Work out the finished part from the listing and answer in its coordinate system (mm). Face numbers are marked on the shaded views. A direction names the side the tool comes from. Give positions to 0.01 mm unless a question says otherwise; leave off trailing zeros. Order: outer loops, then holes, each group sorted by start corner. A loop starts at its lowest first (then second) coordinate and runs counter-clockwise, first axis right, second up. Notation, with made-up numbers: M -17.75,41.25 L 40.25,41.25 A20 cw 40.25,64.25 Z; hole C 44,-31 d2. An arc over 180 degrees is marked long. One line per item, written item: value.
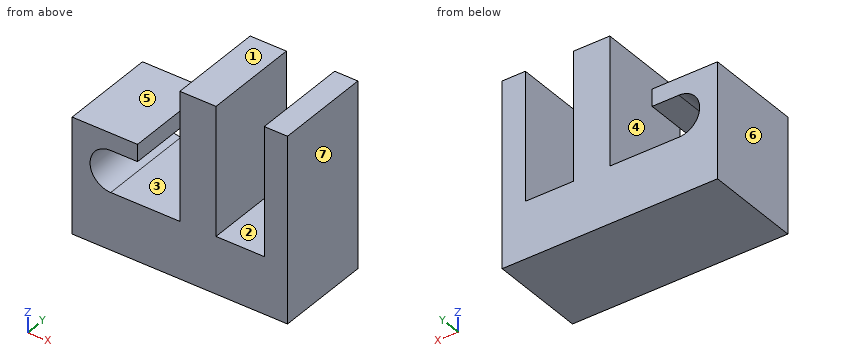
from build123d import *

# Parameters (mm, degrees)
F0_W     = 24.481366
F0_H     = 135.034486
F0_W_2   = 38.1
F0_W_3   = 40.646148
F0_H_2   = 59.899588
F0_H_3   = 43.641134
F0_H_4   = 17.969872
F0_W_4   = 28.23838
F1_DEPTH = 50.8
F3_DEPTH = 176.784


with BuildPart() as f1:
    # F0 (on Front) → F1 (new body, symmetric)
    with BuildSketch(Plane.XZ):
        with Locations((101.140683, 97.467037)):
            Rectangle(F0_W, F0_H)
        with Locations((19.05, 97.467037)):
            Rectangle(F0_W_2, F0_H)
        Polygon((38.1, 29.949794), (0, 29.949794), (-72.735218, 29.949794), (-72.735218, -29.949794), (113.381366, -29.949794), (113.381366, 29.949794), (88.9, 29.949794), align=None)
        with Locations((-93.058292, 0)):
            Rectangle(F0_W_3, F0_H_2)
        with Locations((-93.058292, 51.770361)):
            Rectangle(F0_W_3, F0_H_3)
        with Locations((-93.058292, 82.575864)):
            Rectangle(F0_W_3, F0_H_4)
        with Locations((-58.616028, 82.575864)):
            Rectangle(F0_W_4, F0_H_4)
    extrude(amount=F1_DEPTH, both=True)

    # F2 (on face) → F3 (cut)
    with BuildSketch(Plane.XZ.offset(50.8)):
        with BuildLine():
            Line((-72.735218, 29.949794), (-72.735218, 73.590928))
            ThreePointArc((-72.735218, 73.590928), (-94.555785, 51.770361), (-72.735218, 29.949794))
        make_face()
    extrude(amount=-F3_DEPTH, mode=Mode.SUBTRACT)


solid = f1.part
(1) Section B-B, the plane z = 153 is taken. Give the vertices of the cut face in (x, y).
Findings:
outline: M 0,-50.8 L 38.1,-50.8 L 38.1,50.8 L 0,50.8 Z; M 88.9,-50.8 L 113.38,-50.8 L 113.38,50.8 L 88.9,50.8 Z
(2) Determine the mould class of the marked faces 4, 5, 6 and 7 for opening direction X: pulls with the +X half, pulls with the -X half, needs draft (parallel to the pull), parting line crosses it, or undercut.
Findings:
face 4: undercut
face 5: needs draft
face 6: pulls with the -X half
face 7: pulls with the +X half
(3) Given P1, Ø1.5, axis at x = -26, y = -11, coming from the +Z side, flat-ended and moving along its own axis, determine where the tip first touches the part or whether it passes through.
Findings:
P1: stops at z = 29.95
(4) Find the intervals of material crossed by probe 1 along X at (y, z) = (-37.5, 156.5); probe 2 along X at (y, z) = (-37, 84.5); probe 3 along X at (y, z) = (-9.5, 49.5), in increasing order. Write a range as from..to.
Findings:
probe 1: x = 0..38.1, 88.9..113.38
probe 2: x = -113.38..-44.5, 0..38.1, 88.9..113.38
probe 3: x = -113.38..-94.44, 0..38.1, 88.9..113.38
(5) Section D-D, the plane y = 37.5 is taken. Give the vertices of the cut face in (x, z).
Findings:
outline: M -113.38,-29.95 L 113.38,-29.95 L 113.38,164.98 L 88.9,164.98 L 88.9,29.95 L 38.1,29.95 L 38.1,164.98 L 0,164.98 L 0,29.95 L -72.74,29.95 A21.82 cw -72.74,73.59 L -44.5,73.59 L -44.5,91.56 L -113.38,91.56 Z
(6) Section A-A, the plane x = -63.5 is taken. Give the vertices of the cut face in (y, z), then the cut area to 3 significant figures.
Findings:
outline: M -50.8,-29.95 L 50.8,-29.95 L 50.8,29.95 L -50.8,29.95 Z; M -50.8,73.59 L 50.8,73.59 L 50.8,91.56 L -50.8,91.56 Z
area: 7,910 mm^2
(7) Section C-C, the plane z = 63.5 is taken. Give the vertices of the cut face in (x, y).
Findings:
outline: M -113.38,-50.8 L -91.14,-50.8 L -91.14,50.8 L -113.38,50.8 Z; M 0,-50.8 L 38.1,-50.8 L 38.1,50.8 L 0,50.8 Z; M 88.9,-50.8 L 113.38,-50.8 L 113.38,50.8 L 88.9,50.8 Z
(8) Which of the six approach directions +Z, -Z, +X, -X, +Y, -Y give full straight-line access (tool end or side, diameter ignored) to the marked faces 1, 2 and 3?
Findings:
face 1: +Z, +X, -X, +Y, -Y
face 2: +Z, +Y, -Y
face 3: +Y, -Y
